```python
from build123d import *

# Parameters (mm, degrees)
SKETCH_R     = 2
PAD_DEPTH    = 3
SKETCH001_W  = 4.15
SKETCH001_H  = 90
PAD001_DEPTH = 11.7
SKETCH002_R  = 2
SKETCH002_W  = 50
SKETCH002_H  = 6
POCKET_DEPTH = 15
SKETCH003_W  = 4.09
SKETCH003_H  = 90
PAD002_DEPTH = 3.5
FILLET_R     = 3


with BuildPart() as part:
    # Sketch → Pad (new body)
    with BuildSketch(Plane.XY):
        with BuildLine():
            Line((-14.5, 45), (14.5, 45))
            ThreePointArc((17.5, 42), (16.62132, 44.12132), (14.5, 45))
            Line((17.5, 42), (17.5, 33))
            ThreePointArc((14.5, 30), (16.62132, 30.87868), (17.5, 33))
            Line((14.5, 30), (5, 30))
            Line((5, 30), (5, -30))
            Line((5, -30), (14.5, -30))
            ThreePointArc((17.5, -33), (16.62132, -30.87868), (14.5, -30))
            Line((17.5, -33), (17.5, -42))
            ThreePointArc((14.5, -45), (16.62132, -44.12132), (17.5, -42))
            Line((14.5, -45), (-14.5, -45))
            ThreePointArc((-17.5, -42), (-16.62132, -44.12132), (-14.5, -45))
            Line((-17.5, -42), (-17.5, -33))
            ThreePointArc((-14.5, -30), (-16.62132, -30.87868), (-17.5, -33))
            Line((-5, -30), (-14.5, -30))
            Line((-5, 30), (-5, -30))
            Line((-14.5, 30), (-5, 30))
            ThreePointArc((-17.5, 33), (-16.62132, 30.87868), (-14.5, 30))
            Line((-17.5, 33), (-17.5, 42))
            ThreePointArc((-14.5, 45), (-16.62132, 44.12132), (-17.5, 42))
        make_face()
        with Locations((-10, 37.5)):
            Circle(SKETCH_R, mode=Mode.SUBTRACT)
        with Locations((10, 37.5)):
            Circle(SKETCH_R, mode=Mode.SUBTRACT)
        with Locations((-10, -37.5)):
            Circle(SKETCH_R, mode=Mode.SUBTRACT)
        with Locations((10, -37.5)):
            Circle(SKETCH_R, mode=Mode.SUBTRACT)
    extrude(amount=PAD_DEPTH)

    # Sketch001 → Pad001 (join)
    with BuildSketch(Plane.XY.offset(3)):
        with Locations((-2.925, 0)):
            Rectangle(SKETCH001_W, SKETCH001_H)
        with Locations((2.925, 0)):
            Rectangle(SKETCH001_W, SKETCH001_H)
    extrude(amount=PAD001_DEPTH)

    # Sketch002 → Pocket (cut)
    with BuildSketch(Plane.YZ.offset(5)):
        with Locations((-31.5, 11.5)):
            Circle(SKETCH002_R)
        with Locations((31.5, 11.5)):
            Circle(SKETCH002_R)
        with Locations((0, 12)):
            Rectangle(SKETCH002_W, SKETCH002_H)
    extrude(amount=-POCKET_DEPTH, mode=Mode.SUBTRACT)

    # Sketch003 → Pad002 (join)
    with BuildSketch(Plane.XY.offset(3)):
        with Locations((0.341939, 0)):
            Rectangle(SKETCH003_W, SKETCH003_H)
    extrude(amount=PAD002_DEPTH)

    # Fillet
    fillet_edges = [part.edges().sort_by_distance(p)[0] for p in [
        (-2.925, -45, 14.7),
        (2.925, -45, 14.7),
        (-2.925, -25, 14.7),
        (2.925, -25, 14.7),
        (-2.925, 25, 14.7),
        (2.925, 25, 14.7),
        (-2.925, 45, 14.7),
        (2.925, 45, 14.7),
    ]]
    fillet(fillet_edges, radius=FILLET_R)


solid = part.part
```
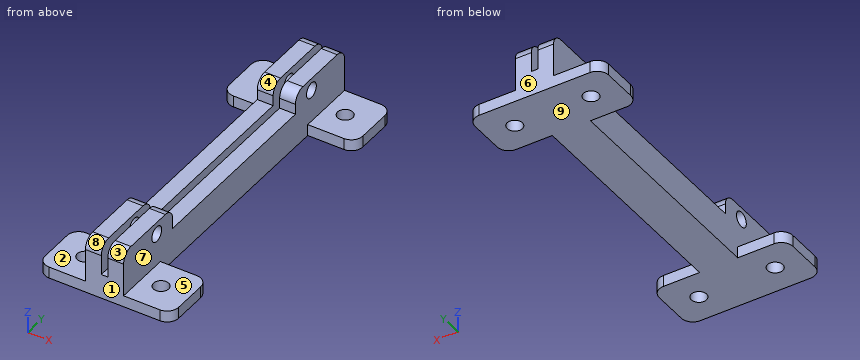
Design review of the part built by this model. Coordinates are the model's own, in mm. Face numbers are marked on the shaded views. A direction names the side the tool comes from. Round coordinates to 2 decimals unless told otherwise and drop trailing zeros. Order: outer loops, then holes, each group sorted by start corner. A loop starts at its lowest first (then second) coordinate and runs counter-clockwise, first axis right, second up. Notation, with made-up numbers: (13, -24.75) - (17, -24.75) arc R5 cw to (17, -16.75) - close; hole circle Ø7 at (12, 54). An arc over 180 degrees is marked (long way). Return JSON: item names as keys, results as strings.
Q1. For pin 1 Ø2 at (y, z) = (28.5, 11) entering from +X; pin 2 Ø6.5 at (y, z) = (1.5, 8.5) entering from -X; pin 3 Ø4.5 at (x, y) = (-3.5, 7) entering from +Z; pin 4 Ø6.5 at (x, y) = (10, 37.5) entering from -Z, all flat-tipped, find the tip position at first contact; note any pin that passes through.
Computed values:
{"pin 1": "stops at x = 5", "pin 2": "stops at x = -5", "pin 3": "stops at z = 9", "pin 4": "stops at z = 0"}
Q2. The part is to be moulded in two halves that separate along Y. For the marked faces 6, 7, 8 and 9, say which applies: pulls with the +Y half, pulls with the -Y half, needs draft (parallel to the pull), parting line crosses it, or undercut.
Computed values:
{"face 6": "pulls with the +Y half", "face 7": "undercut", "face 8": "pulls with the -Y half", "face 9": "needs draft"}
Q3. Consider section A-A on x = -10. Write out the cut boundary in (y, z), plus the area to 3 significant figures.
Computed values:
{"outline": "(-45, 0) - (-39.5, 0) - (-39.5, 3) - (-45, 3) - close; (-35.5, 0) - (-30, 0) - (-30, 3) - (-35.5, 3) - close; (30, 0) - (35.5, 0) - (35.5, 3) - (30, 3) - close; (39.5, 0) - (45, 0) - (45, 3) - (39.5, 3) - close", "area": "66.0 mm2"}
Q4. Machinability: for the marked faces 1, 2, 3, 4 and 5, which of the approach directions +Z, -Z, +X, -X, +Y, -Y give a long, thin tool a straight path to every point of the face, cutting with its end or side? Answer none if there is none.
Computed values:
{"face 1": "+Z, -Z, +X, -X, -Y", "face 2": "+Z, -X, +Y, -Y", "face 3": "+Z, +X, -X, -Y", "face 4": "+Z, +X, -X", "face 5": "+Z, +X, +Y, -Y"}
Q5. Consider section B-B on y = 37.5. Write out the cut boundary in (x, z).
Computed values:
{"outline": "(-17.5, 0) - (-12, 0) - (-12, 3) - (-17.5, 3) - close; (-8, 0) - (8, 0) - (8, 3) - (5, 3) - (5, 14.7) - (0.85, 14.7) - (0.85, 6.5) - (-0.85, 6.5) - (-0.85, 14.7) - (-5, 14.7) - (-5, 3) - (-8, 3) - close; (12, 0) - (17.5, 0) - (17.5, 3) - (12, 3) - close"}
Q6. Consider section C-C on x = 6. Write out the cut boundary in (y, z).
Computed values:
{"outline": "(-45, 0) - (-30, 0) - (-30, 3) - (-45, 3) - close; (30, 0) - (45, 0) - (45, 3) - (30, 3) - close"}
Q7. Consider section D-D on x = -2.5. Write out the cut boundary in (y, z), plus the area to 3 significant figures.
Computed values:
{"outline": "(-45, 0) - (45, 0) - (45, 11.7) arc R3 ccw to (42, 14.7) - (28, 14.7) arc R3 ccw to (25, 11.7) - (25, 9) - (-25, 9) - (-25, 11.7) arc R3 ccw to (-28, 14.7) - (-42, 14.7) arc R3 ccw to (-45, 11.7) - close; hole circle Ø4 at (-31.5, 11.5); hole circle Ø4 at (31.5, 11.5)", "area": "1,010 mm2"}
Q8. Wall thickness on L1, parallel to Y at x = 7, z = 2.5; L2, parallel to X at y = 37, z = 2; L3, parallel to Y at x = -10, z = 2.45: over which ranges is each line inside the solid? List them lowest first. Write a range as [from, to].
Computed values:
{"L1": "y = [-45, -30], [30, 45]", "L2": "x = [-17.5, -11.94], [-8.06, 8.06], [11.94, 17.5]", "L3": "y = [-45, -39.5], [-35.5, -30], [30, 35.5], [39.5, 45]"}
